Can you work these out from the drawing? Everything is in mm from the part's minimum corner. Give positions to 0.01 mm unless a question says otherwise; leave off trailing zeros. Order: outer loops, then holes, each group sorted by start corner. A loop starts at its lowest first (then second) coordinate and runs counter-clockwise, first axis right, second up. Notation, with made-up numbers: (73.5, 69.5) - (102.5, 69.5) arc R19 ccw to (102.5, 101.5) - close; hole circle Ø5 at (8, -39). An arc over 180 degrees is marked (long way). Answer as a JSON object with one key per item and string values.
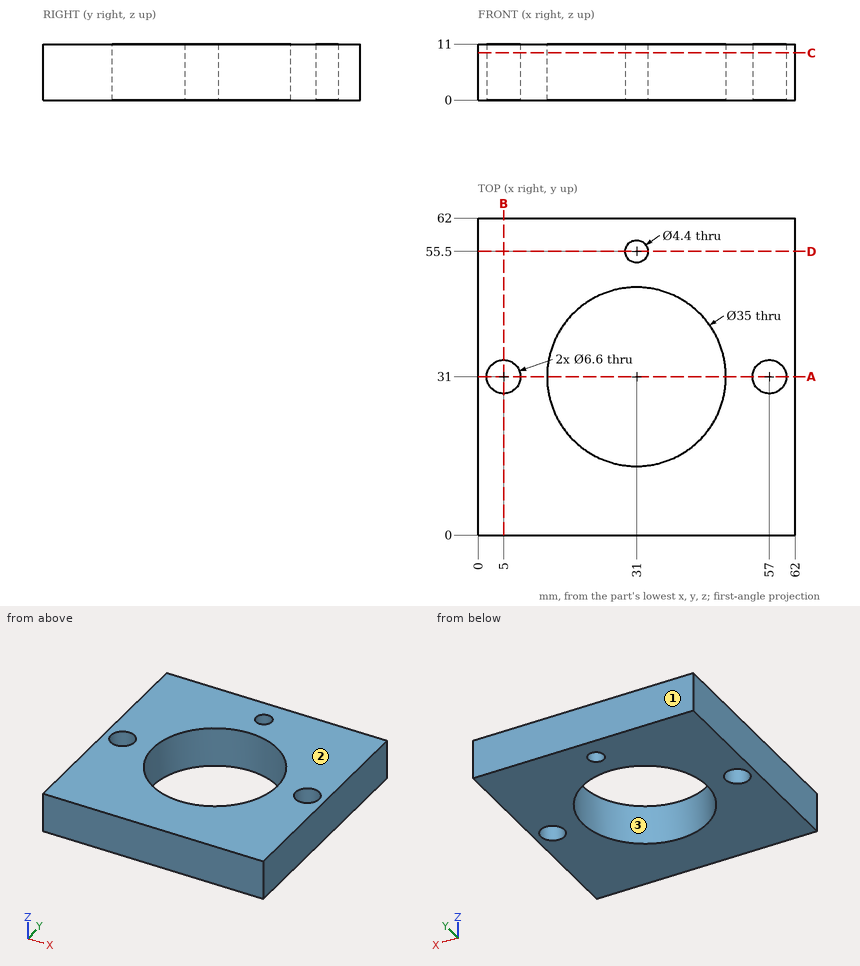
Q1. If we section it at D-D, the plane y = 55.5: Please give me the cut outline in (x, z), then the cut area to 3 significant figures.
Recorded:
{"outline": "(0, 0) - (28.8, 0) - (28.8, 11) - (0, 11) - close; (33.2, 0) - (62, 0) - (62, 11) - (33.2, 11) - close", "area": "634 mm^2"}
Q2. If we section it at A-A, the plane y = 31: Please give me the cut outline in (x, z), then the cut area to 3 significant figures.
Recorded:
{"outline": "(0, 0) - (1.7, 0) - (1.7, 11) - (0, 11) - close; (8.3, 0) - (13.5, 0) - (13.5, 11) - (8.3, 11) - close; (48.5, 0) - (53.7, 0) - (53.7, 11) - (48.5, 11) - close; (60.3, 0) - (62, 0) - (62, 11) - (60.3, 11) - close", "area": "152 mm^2"}
Q3. If we section it at C-C, the plane z = 9.25: Please give me the cut outline in (x, y), then the cut area to 3 significant figures.
Recorded:
{"outline": "(0, 0) - (62, 0) - (62, 62) - (0, 62) - close; hole circle Ø6.6 at (5, 31); hole circle Ø35 at (31, 31); hole circle Ø4.4 at (31, 55.5); hole circle Ø6.6 at (57, 31)", "area": "2,800 mm^2"}
Q4. If we section it at B-B, the plane x = 5: Please give me the cut outline in (y, z), then the cut area to 3 significant figures.
Recorded:
{"outline": "(0, 0) - (27.7, 0) - (27.7, 11) - (0, 11) - close; (34.3, 0) - (62, 0) - (62, 11) - (34.3, 11) - close", "area": "609 mm^2"}
Q5. I need wall thicknesses on L1, parallel to Y at x = 31, z = 5.75; L2, parallel to Y at x = 57, z = 3; L3, parallel to X at y = 30, z = 8.75. Which ranges of each line are inside material? Lowest first, please.
Recorded:
{"L1": "y = 0 to 13.5, 48.5 to 53.3, 57.7 to 62", "L2": "y = 0 to 27.7, 34.3 to 62", "L3": "x = 0 to 1.86, 8.14 to 13.53, 48.47 to 53.86, 60.14 to 62"}
Q6. We'd pull the mould along Y, two halves only. Please class the marked faces 1, 2 and 3: released by +Y, released by -Y, zero draft, split by the parting line, or undercut.
Recorded:
{"face 1": "released by +Y", "face 2": "zero draft", "face 3": "undercut"}
Q7. I'm going to push a flat-ended pin straight in: pin 1 Ø6 at (x, y) = (57, 31) entering from +Z. Where does the tip first touch, or does it pass through?
Recorded:
{"pin 1": "passes through"}
